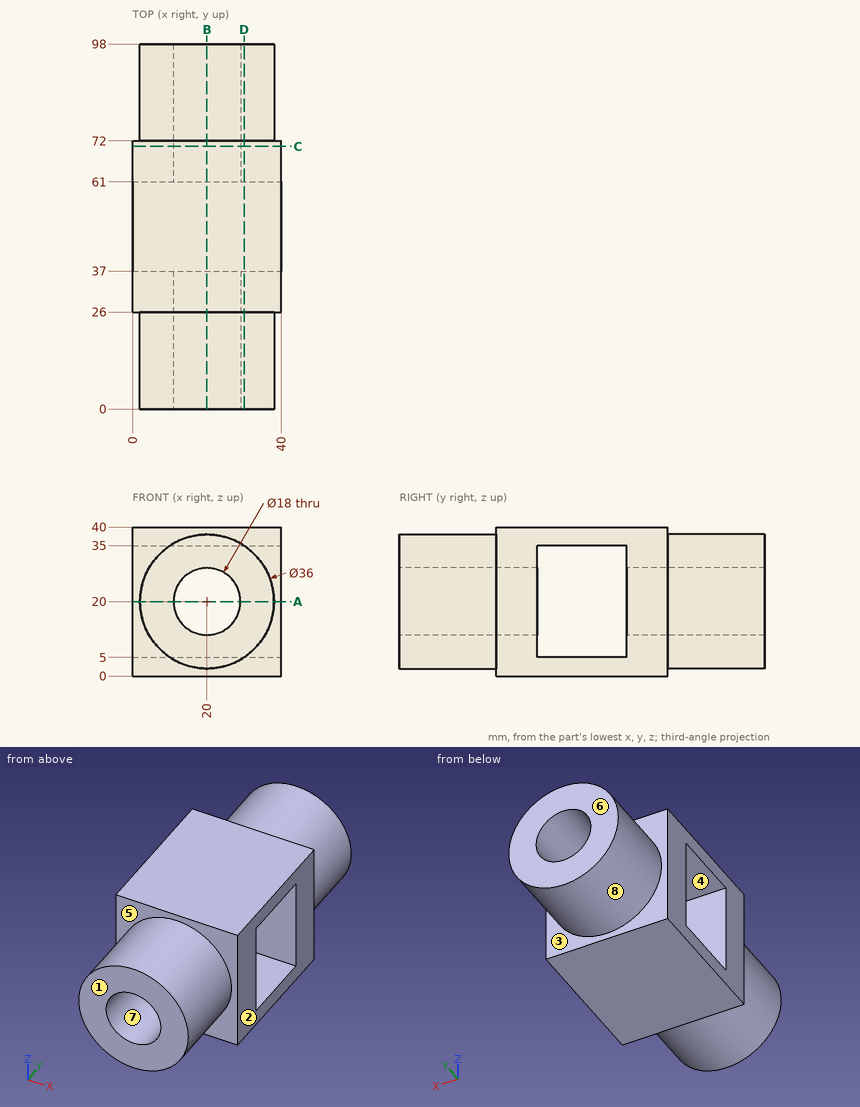
Geometry: see drawing. Coordinates: mm, zero at the bounding-box minimum. A direction names the side the tool comes from. Give positions to 0.01 mm unless a question says otherwise; leave off trailing zeros. Loops run counter-clockwise (first coordinate to the right, second up) from the corner with the lowest first, then second, coordinate; pieces in that order, holes last. Notation, with made-up numbers: (5.25, 51) -> (55.25, 51) arc R11 cw to (55.25, 59) -> close; hole circle Ø6 at (33.25, 29.25). An arc over 180 degrees is marked (long way). Use one line per item in the form item = value.
Item 1: Pin query (flat end, axial travel): P1, Ø2, axis at x = 10.5, y = 21.5, coming from the -Z side. Return the tip coordinate at first contact, or that it passes through.
A:
P1 = 4.13
Item 2: Access query for the marked faces 1, 2, 3, 4 and 5. Directions: +Z, -Z, +X, -X, +Y, -Y. A direction counts if a zero-diameter tool reaches every point of the face in a straight line with its end or side. Return the directions, or none.
A:
face_1 = +Z, -Z, +X, -X, -Y
face_2 = +Z, -Z, +X, +Y, -Y
face_3 = +Y
face_4 = +X, -X
face_5 = -Y
Item 3: Section query C-C on y = 70.5. Output: boundary loops of the cut face in (x, z).
A:
outline = (0, 0) -> (40, 0) -> (40, 40) -> (0, 40) -> close; hole circle Ø18 at (20, 20)
Item 4: Section query A-A on z = 20. Output: boundary loops of the cut face in (x, y), and give its area (3 significant figures).
A:
outline = (0, 26) -> (2, 26) -> (2, 0) -> (11, 0) -> (11, 37) -> (0, 37) -> close; (0, 61) -> (11, 61) -> (11, 98) -> (2, 98) -> (2, 72) -> (0, 72) -> close; (29, 0) -> (38, 0) -> (38, 26) -> (40, 26) -> (40, 37) -> (29, 37) -> close; (29, 61) -> (40, 61) -> (40, 72) -> (38, 72) -> (38, 98) -> (29, 98) -> close
area = 1,420 mm^2
Item 5: Draft query along X for the marked faces 6, 7 and 8. Return one class per face: pulls with the +X half, pulls with the -X half, needs draft (parallel to the pull), parting line crosses it, or undercut.
A:
face_6 = needs draft
face_7 = undercut
face_8 = parting line crosses it
Item 6: Line query: probe 1 along Z at (x, y) = (20, 86); probe 2 along Z at (x, y) = (30, 59.5); probe 3 along Y at (x, z) = (29.5, 12). Output: solid intervals per line, ascending.
A:
probe_1 = 2 to 11, 29 to 38
probe_2 = 0 to 5, 35 to 40
probe_3 = 0 to 37, 61 to 98
Item 7: Section query B-B on x = 20. Output: boundary loops of the cut face in (y, z).
A:
outline = (0, 2) -> (26, 2) -> (26, 0) -> (72, 0) -> (72, 2) -> (98, 2) -> (98, 11) -> (61, 11) -> (61, 5) -> (37, 5) -> (37, 11) -> (0, 11) -> close; (0, 29) -> (37, 29) -> (37, 35) -> (61, 35) -> (61, 29) -> (98, 29) -> (98, 38) -> (72, 38) -> (72, 40) -> (26, 40) -> (26, 38) -> (0, 38) -> close
Item 8: Section query D-D on x = 30. Output: boundary loops of the cut face in (y, z), and give its area (3 significant figures).
A:
outline = (0, 5.03) -> (26, 5.03) -> (26, 0) -> (72, 0) -> (72, 5.03) -> (98, 5.03) -> (98, 34.97) -> (72, 34.97) -> (72, 40) -> (26, 40) -> (26, 34.97) -> (0, 34.97) -> close; hole (37, 5) -> (61, 5) -> (61, 35) -> (37, 35) -> close
area = 2,680 mm^2
